Build history of the part. All positions in model axes, mm. A direction names the side the tool comes from. Coordinates: 2 decimals unless noted, no trailing zeros. Write each loop counter-clockwise with the first axis right and the second up, starting at its lowest first coordinate (ties: lowest second). Pieces come first, ordered by that corner, then holes.
```python
from build123d import *

# Parameters (mm, degrees)
F1_DEPTH = 80
F2_T     = -5


with BuildPart() as f1:
    # F0 (on Front) → F1 (new body)
    with BuildSketch(Plane.XZ):
        with BuildLine():
            Line((-348.8748669624, 349.0544557571), (-198.1384754181, -82.8632265329))
            Line((-198.1384754181, -82.8632265329), (212.5215083361, -82.8632265329))
            Line((212.5215083361, -82.8632265329), (356.4940690994, 346.1556732655))
            Line((356.4940690994, 346.1556732655), (145.8496451378, 136.4775151014))
            ThreePointArc((145.8496451378, 136.4775151014), (107.5303186219, 45.3719417758), (107.1992963552, 144.2075967789))
            Line((107.1992963552, 144.2075967789), (0, 427.7250468731))
            Line((0, 427.7250468731), (-97.6475700736, 143.2413309813))
            ThreePointArc((-97.6475700736, 143.2413309813), (-100.1659657794, 46.0677822233), (-138.2304430008, 135.511264205))
            Line((-138.2304430008, 135.511264205), (-348.8748669624, 349.0544557571))
        make_face()
        with BuildLine():
            ThreePointArc((-4.4474751757, 7.729579965), (-2.6813223644, 20.5003556429), (8.1768609292, 13.5496820978))
            ThreePointArc((8.1768609292, 13.5496820978), (7.5196984972, 10.4468328198), (5.6610608526, 7.8768129348))
            Line((5.6610608526, 7.8768129348), (9.4852344756, -7.0666760483))
            Line((9.4852344756, -7.0666760483), (-8.1122881109, -7.0666760483))
            Line((-8.1122881109, -7.0666760483), (-4.4474751757, 7.729579965))
        make_face(mode=Mode.SUBTRACT)
    extrude(amount=F1_DEPTH)

    # F2
    f2_openings = [f1.faces().sort_by_distance(p)[0] for p in [
        (6.021536, 0, 100.900986),
    ]]
    offset(amount=F2_T, openings=f2_openings, kind=Kind.INTERSECTION)


solid = f1.part
```
1. Mould opens along Z. For faces 4 (the face through (-98.317, -39.44, 46.456)), 5 (the face through (-1, -80, 119)), 6 (the face through (-266.71, -36.98, 128.79)), 7 (the face through (283.5, -39.44, 128.64)) say: +Z half, -Z half, draft (parallel to the pull), parting line (faces both ways), or undercut.
Computed values:
face 4: undercut
face 5: draft
face 6: undercut
face 7: -Z half
2. Flat gauge pins, fed straight in: pin 1 (4 mm diameter, centred on y = -53, z = 50.5, fed in from +X); pin 2 (6 mm diameter, centred on x = -127.5, y = -37, fed in from +Z); pin 3 (4 mm diameter, centred on x = -22, z = 76, fed in from +Y). Where does each tip first touch, or does it go through?
Computed values:
pin 1: stops at x = 257.95
pin 2: stops at z = 49.85
pin 3: stops at y = -75
3. Saw through at C-C on x = -23. List the corners of the cut face in (y, z).
Computed values:
outline: (-80, -82.86) - (0, -82.86) - (0, -77.86) - (-75, -77.86) - (-75, 345.32) - (0, 345.32) - (0, 360.72) - (-80, 360.72) - close
4. Saw through at A-A on y = -17.5. List the corners of the cut face in (x, z), plus the area to 3 significant figures.
Computed values:
outline: (-348.87, 349.05) - (-198.14, -82.86) - (212.52, -82.86) - (356.49, 346.16) - (145.85, 136.48) arc R50.43 cw (long way) to (107.2, 144.21) - (0, 427.73) - (-97.65, 143.24) arc R49.74 cw (long way) to (-138.23, 135.51) - close; (-14.5, -12.07) - (15.93, -12.07) - (11.13, 6.66) arc R12.65 ccw (long way) to (-9.93, 6.41) - close; hole (-336.83, 329.73) - (-194.59, -77.86) - (208.93, -77.86) - (345.02, 327.68) - (153.43, 136.97) arc R55.43 cw (long way) to (100.56, 147.63) - (0.23, 412.99) - (-91.23, 146.54) arc R54.74 cw (long way) to (-145.7, 135.96) - close; hole (-8.11, -7.07) - (9.49, -7.07) - (5.66, 7.88) arc R7.65 ccw (long way) to (-4.45, 7.73) - close
area: 15,600 mm2
5. 3-axis set-ups, long thin cutter, end or side, ignore diameter. For faces 1 (the face through (109.43, -39.44, 45.03)), 2 (the face through (250.565, -36.975, 233.658)), 3 (the face through (252.646, -39.44, 242.784)): which of +Z, -Z, +X, -X, +Y, -Y reach the whole face in a straight line?
Computed values:
face 1: +Y, -Y
face 2: +Y
face 3: +Z, +Y, -Y
6. Probe line 1 along X through (y, z) = (-32, 22); line 2 along X through (y, z) = (-70, 128); line 3 along X through (y, z) = (-68, 303). List the from-to ranges inside material, lowest first.
Computed values:
line 1: x = -234.74 to -229.44, -8.9 to 9.94, 242.44 to 247.71
line 2: x = -271.73 to -266.43, -153.09 to -146.62, -72.32 to -65.85, 73.01 to 79.44, 155.4 to 161.83, 278.01 to 283.28
line 3: x = -332.8 to -327.51, -310.47 to -303.45, -42.81 to -37.52, 41.81 to 47.16, 313.14 to 320.23, 336.74 to 342.01
7. Saw through at D-D on z = -45.5. List the corners of the cut face in (x, y), plus the area to 3 significant figures.
Computed values:
outline: (-211.18, -80) - (225.06, -80) - (225.06, 0) - (219.79, 0) - (219.79, -75) - (-205.88, -75) - (-205.88, 0) - (-211.18, 0) - close
area: 2,970 mm2
8. Saw through at B-B on z = 158. List the corners of the cut face in (x, y).
Computed values:
outline: (-282.2, -80) - (-160.41, -80) - (-160.41, 0) - (-167.44, 0) - (-167.44, -75) - (-276.9, -75) - (-276.9, 0) - (-282.2, 0) - close; (-92.58, -80) - (101.98, -80) - (101.98, 0) - (96.64, 0) - (96.64, -75) - (-87.3, -75) - (-87.3, 0) - (-92.58, 0) - close; (167.47, -80) - (293.35, -80) - (293.35, 0) - (288.08, 0) - (288.08, -75) - (174.56, -75) - (174.56, 0) - (167.47, 0) - close
